Autodesk Inventor part; units mm, degrees
ref_plane "MSC_PF1" through (0, 0, 0) normal (1, 0, 0) x (0, 1, 0)
ref_plane "MSC_PT1" through (0, 0, 0) normal (0, 0, -1) x (-1, 0, 0)
ref_plane "YZ Plane" through (0, 0, 0) normal (1, 0, 0) x (0, 1, 0)
sketch "Esquisse1" plane through (0, 0, 0) normal (0, 1, 0) x (-1, 0, 0)
  point P0 (0, 0)
sketch "Esquisse2" plane through (0, 0, 0) normal (0, 0, 1) x (1, 0, 0)
  point P0 (0, 0)
sketch "Esquisse3" plane through (0, 0, 0) normal (0, 0, 1) x (1, 0, 0)
  point P0 (0, 0)
sketch "Esquisse4" plane through (0, 0, 0) normal (0, 1, 0) x (-1, 0, 0)
  line L0 (-2.75, 0) -> (0, 0)
  line L1 (-2.75, -0.4) -> (-2.75, 0)
  line L2 (-1.5, -1.65) -> (-2.75, -0.4)
  line L3 (-1.5, -1.9) -> (-1.5, -1.65)
  line L4 (-1.25, -2.15) -> (-1.5, -1.9)
  line L5 (-1.5, -2.4) -> (-1.25, -2.15)
  line L6 (-1.5, -4) -> (-1.5, -2.4)
  line L7 (0, 0) -> (0, -4)
  line L8 (0, 3.3392) -> (0, -10.7) construction
  line L9 (0, 3.3392) -> (0, -10.7)
  line L10 (0, -13.5078) -> (0, 6.1471)
  line L11 (-1.5, -4) -> (0, -4)
  line L12 (0.55, 0) -> (-3.3, 0)
  dimension "d3" = 2.75
  dimension "d5" = 0.25
  dimension "d7" = 0.25
  dimension "d9" = 0.25
  dimension "d11" = 1.65
  dimension "d13" = 135
  dimension "d17" = 1.25
  dimension "d19" = 0
  dimension "d51" = 1.5
  dimension "d52" = 4
revolve "Révolution1" add sketch "Esquisse4" angle 360 about axis through (0, 0, 3.3392) along (0, 0, -1)
sketch "Esquisse5" plane through (0, 0, 0) normal (0, 1, 0) x (-1, 0, 0)
  line L0 (-1.6, 0) -> (0, 0)
  line L1 (-0.2667, -1.5) -> (-1.6, 0)
  line L2 (0, -1.5) -> (-0.2667, -1.5)
  line L3 (0, 0) -> (0, -1.5)
  line L4 (-1.5, -1.65) -> (1.5, -1.65) construction
  line L5 (-2.75, 0) -> (2.75, 0)
  line L6 (0, -1.98) -> (0, 0.33)
  dimension "d22" = 1.6
  dimension "d24" = 0.2667
  dimension "d26" = 1.5
extrude "Extrusion1" cut sketch "Esquisse5" along normal mid plane 0.5333
pattern_circular "RéseauPolaire1" count 4 over 360 about axis through (0, 0, 0) along (0, 0, 1) of "Extrusion1"
sketch "Esquisse7" plane through (0, 0, 0) normal (0, 1, 0) x (-1, 0, 0)
  line L0 (0, -0.825) -> (-2, 0)
  line L1 (0, 0) -> (0, -0.825)
  line L2 (-2, 0) -> (0, 0)
  line L3 (-1.5, -1.65) -> (1.5, -1.65) construction
  line L4 (0, -1.98) -> (0, 0.33)
  line L5 (-2.75, 0) -> (2.75, 0)
  dimension "d33" = 2
  dimension "d35" = 0.825
extrude "Extrusion2" cut sketch "Esquisse7" along normal mid plane 0.5333
pattern_circular "RéseauPolaire2" count 4 over 360 about axis through (0, 0, 0) along (0, 0, 1) of "Extrusion2"
fillet "Congé1" radius 0.5 1 edges at (-1.5, 0, -1.65)
thread "Filetage1"
ref_plane "MSC_PF1" through (0, 0, 0) normal (1, 0, 0) x (0, 1, 0)
ref_plane "MSC_PT1" through (0, 0, 0) normal (0, 0, -1) x (-1, 0, 0)
equation "\"d3\" = 0.5 * Dh"
equation "\"d5\" = msp_x"
equation "\"d7\" = ParA"
equation "\"d9\" = msp_x"
equation "\"d11\" = ParK"
equation "\"d17\" = 0.5 * msp_mdtds"
equation "\"d51\" = 0.5 * NND"
equation "\"d52\" = NLG"
equation "\"d22\" = 0.5 * M"
equation "\"d24\" = 0.0833333 * M"
equation "\"d26\" = 0.909091 * ParK"
equation "\"d27\" = 0.166667 * M"
equation "\"d33\" = 0.625 * M"
equation "\"d35\" = 0.5 * ParK"
equation "\"d36\" = 0.166667 * M"
equation "\"d41\" = 2 * msp_x"
equation "\"PTC\" = 0.5"
equation "\"NLG\" = 4"
equation "\"ParK\" = 1.65"
equation "\"NND\" = 3"
equation "\"M\" = 3.2"
equation "\"msp_mdtds\" = NND - PTC"
equation "\"Dh\" = 5.5"
equation "\"msp_x\" = 0.5 * PTC"
equation "\"ParA\" = 0.5 * PTC"
equation "\"r\" = 0.8"
equation "\"THREADDIA\" = NND"
equation "\"TEMPLATE\" = 1.2345"
properties part number "NF EN ISO 7046-2 H - M3x4 - 8.8 - H1" material "Acier inoxydable 440C"
Verification items for the finished model (mm, model axes). A direction names the side the tool comes from. Coordinates: 2 decimals unless noted, no trailing zeros. Write each loop counter-clockwise with the first axis right and the second up, starting at its lowest first coordinate (ties: lowest second). Pieces come first, ordered by that corner, then holes. Notation, with made-up numbers: M 53.5,22 L 67.5,22 A11 ccw 67.5,34 Z; hole C 83.5,-15.75 d10. An arc over 180 degrees is marked long. Use a Markdown table: item, result.
Q1. Sectioned sample at C-C, the plane z = -1.4. Record the boundary of the cut face in (x, y), plus the area to 3 significant figures.
Reply:
| item | result |
|---|---|
| outline | C 0,0 d3.5; hole M -0.36,-0.27 L -0.27,-0.27 L -0.27,-0.36 L 0.27,-0.36 L 0.27,-0.27 L 0.36,-0.27 L 0.36,0.27 L 0.27,0.27 L 0.27,0.36 L -0.27,0.36 L -0.27,0.27 L -0.36,0.27 Z |
| area | 9.15 mm² |
Q2. Set-up check for faces 4 (the face through (0.8, 0, -0.9)), 5 (the face through (-0.596, -2.685, -0.197)): record each of +Z, -Z, +X, -X, +Y, -Y from which the full face is reachable in a straight line by a thin tool's end or side.
Reply:
| item | result |
|---|---|
| face 4 | +Z |
| face 5 | +Z, -Z |
Q3. Draft check along X on faces 1 (the face through (0, 0, -4)), 2 (the face through (0, -0.8, -0.9)), 3 (the face through (-1.5, 0.07, -3.19)). Enter one of: +X half, -X half, draft (parallel to the pull), parting line (faces both ways), or undercut.
Reply:
| item | result |
|---|---|
| face 1 | draft |
| face 2 | undercut |
| face 3 | parting line |
Q4. Sectioned sample at A-A, the plane z = -0.9. Record the boundary of the cut face in (x, y), plus the area to 3 significant figures.
Reply:
| item | result |
|---|---|
| outline | C 0,0 d4.5; hole M -0.8,-0.27 L -0.27,-0.27 L -0.27,-0.8 L 0.27,-0.8 L 0.27,-0.27 L 0.8,-0.27 L 0.8,0.27 L 0.27,0.27 L 0.27,0.8 L -0.27,0.8 L -0.27,0.27 L -0.8,0.27 Z |
| area | 14.5 mm² |
Q5. Thickness scan on line 1 (Y direction, x = 0.45, z = -0.2); line 2 (Y direction, x = -0.4, z = -1.05); line 3 (X direction, y = 0.2, z = -1.05). Record the ranges inside material, lowest first.
Reply:
| item | result |
|---|---|
| line 1 | y = -2.71 to -0.27, 0.27 to 2.71 |
| line 2 | y = -2.06 to -0.27, 0.27 to 2.06 |
| line 3 | x = -2.09 to -0.67, 0.67 to 2.09 |
Q6. Sectioned sample at B-B, the plane z = -2.25. Record the boundary of the cut face in (x, y), plus the area to 3 significant figures.
Reply:
| item | result |
|---|---|
| outline | C 0,0 d2.7 |
| area | 5.73 mm² |
Q7. Go/stop test with flat-tipped pins: P1, Ø0.5, axis at y = 1.5, z = -1, coming from the -X side; P2, Ø0.8, axis at y = -1.5, z = -0.5, coming from the +X side; P3, Ø1.7, axis at x = -1, z = -1, coming from the -Y side. Record where each tip stops, or that it passes through.
Reply:
| item | result |
|---|---|
| P1 | stops at x = -1.93 |
| P2 | stops at x = 2.51 |
| P3 | stops at y = -2.72 |
